Verification items for the finished model (mm, model axes). Face numbers are marked on the shaded views. Coordinates: 2 decimals unless noted, no trailing zeros. Write each loop counter-clockwise with the first axis right and the second up, starting at its lowest first coordinate (ties: lowest second). Pieces come first, ordered by that corner, then holes.
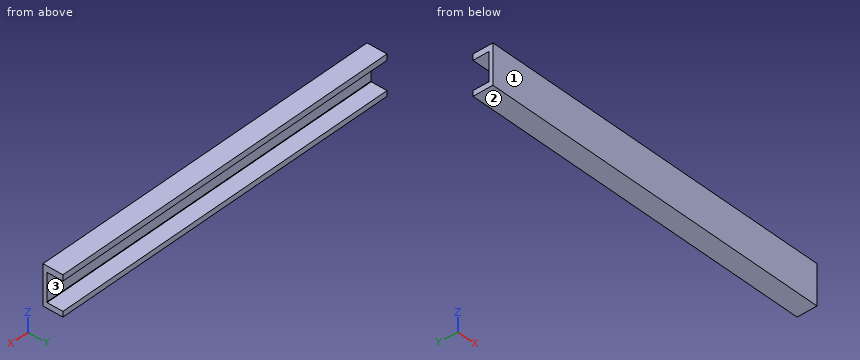
```python
from build123d import *

# Parameters (mm, degrees)
ESQUISSE1_W             = 1800
ESQUISSE1_H             = 100
BOSS_EXTRU_1_DEPTH      = 200
ESQUISSE2_W             = 1800
ESQUISSE2_H             = 140
ENL_V_MAT_EXTRU_1_DEPTH = 80
ESQUISSE4_W             = 1800
ESQUISSE4_H             = 2.941473276
ENL_V_MAT_EXTRU_2_DEPTH = 79.5


with BuildPart() as part:
    # Esquisse1 → Boss.-Extru.1 (new body)
    with BuildSketch(Plane.XY):
        with Locations((0, -50)):
            Rectangle(ESQUISSE1_W, ESQUISSE1_H)
    extrude(amount=BOSS_EXTRU_1_DEPTH)

    # Esquisse2 → Enlèv. mat.-Extru.1 (cut)
    with BuildSketch(Plane(origin=(0, 0, 0), x_dir=(1, 0, 0), z_dir=(0, 1, 0))):
        with Locations((0, -100)):
            Rectangle(ESQUISSE2_W, ESQUISSE2_H)
    extrude(amount=-ENL_V_MAT_EXTRU_1_DEPTH, mode=Mode.SUBTRACT)

    # Esquisse4 → Enlèv. mat.-Extru.2 (cut)
    with BuildSketch(Plane(origin=(0, 0, 0), x_dir=(1, 0, 0), z_dir=(0, 1, 0))):
        with Locations((0, -28.529263362)):
            Rectangle(ESQUISSE4_W, ESQUISSE4_H)
    extrude(amount=-ENL_V_MAT_EXTRU_2_DEPTH, mode=Mode.SUBTRACT)


solid = part.part
```
1. Material ranges on L1, parallel to Z at x = 794.5, y = -23.5; L2, parallel to Y at x = -226, z = 124.5; L3, parallel to Y at x = 430, z = 29.5, recorded low to high.
2. Sectioned sample at B-B, the plane x = -652. Record the boundary of the cut face in (y, z).
3. Draft check along Z on the marked faces 1, 2 and 3. Enter one of: pulls with the +Z half, pulls with the -Z half, needs draft (parallel to the pull), parting line crosses it, or undercut.
4. Sectioned sample at A-A, the plane y = -37.5. Record the boundary of the cut face in (x, z), and give its area (3 significant figures).
5. Gauge pin test, flat ends, axial feed: P1, Ø3, axis at x = -367, z = 29, coming from the +Y side; P2, Ø1.5, axis at x = 460.5, z = 77, coming from the +Y side. Record the tip position at first contact, or that the pin passes through.
6. Sectioned sample at C-C, the plane z = 72. Record the boundary of the cut face in (x, y).
Outcome:
1. L1: z = 0 to 27.06, 170 to 200
1. L2: y = -100 to -80
1. L3: y = -100 to -79.5
2. outline: (-100, 0) - (0, 0) - (0, 27.06) - (-79.5, 27.06) - (-79.5, 30) - (-80, 30) - (-80, 170) - (0, 170) - (0, 200) - (-100, 200) - close
3. face 1: needs draft
3. face 2: pulls with the -Z half
3. face 3: undercut
4. outline: (-900, 0) - (900, 0) - (900, 27.06) - (-900, 27.06) - close; (-900, 170) - (900, 170) - (900, 200) - (-900, 200) - close
4. area: 103,000 mm2
5. P1: stops at y = -79.5
5. P2: stops at y = -80
6. outline: (-900, -100) - (900, -100) - (900, -80) - (-900, -80) - close
